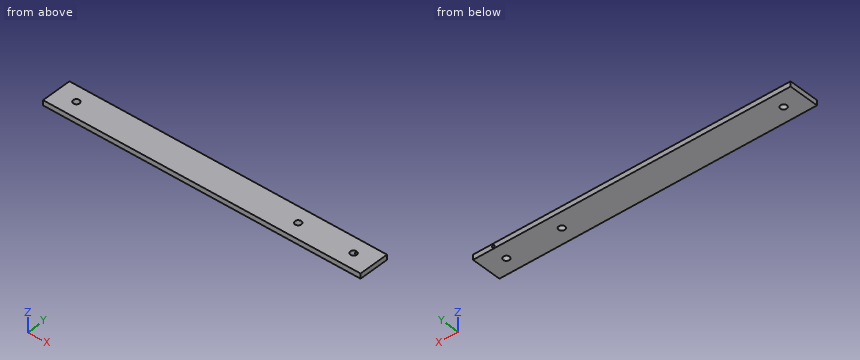
from build123d import *

# Parameters (mm, degrees)
SKETCH1_W               = 800.1
SKETCH1_H               = 76.2
BOSS_EXTRUDE1_DEPTH     = 12.7
CUT_EXTRUDE1_DEPTH      = 611.921484317
CUT_EXTRUDE1_DEPTH_BACK = 611.921484317
SKETCH2_R               = 7.9375
CUT_EXTRUDE2_DEPTH      = 615.475296493
CUT_EXTRUDE2_DEPTH_BACK = 31.75
SKETCH3_R               = 3.175


with BuildPart() as part:
    # Sketch1 → Boss-Extrude1 (new body)
    with BuildSketch(Plane.XY):
        with Locations((-209.55, 0)):
            Rectangle(SKETCH1_W, SKETCH1_H)
    extrude(amount=BOSS_EXTRUDE1_DEPTH)

    # Sketch2 → Cut-Extrude1 (cut, two sides: drawn at the far end of the back side and taken through both)
    with BuildSketch(Plane.XY.offset(12.7).offset(-CUT_EXTRUDE1_DEPTH_BACK)):
        Circle(SKETCH2_R)
        with Locations((-558.8, 0)):
            Circle(SKETCH2_R)
        with Locations((139.7, 0)):
            Circle(SKETCH2_R)
    extrude(amount=CUT_EXTRUDE1_DEPTH + CUT_EXTRUDE1_DEPTH_BACK, mode=Mode.SUBTRACT)

    # Sketch3 → Cut-Extrude2 (cut, two sides: drawn at the far end of the back side and taken through both)
    with BuildSketch(Plane(origin=(0, 38.1, 0), x_dir=(1, 0, 0), z_dir=(0, 1, 0)).offset(-CUT_EXTRUDE2_DEPTH_BACK)):
        with Locations(Location((139.7, -6.212362636, 0), (0, 0, 90))):
            Circle(SKETCH3_R)
    extrude(amount=CUT_EXTRUDE2_DEPTH + CUT_EXTRUDE2_DEPTH_BACK, mode=Mode.SUBTRACT)


solid = part.part
Could you check a few things on this model? Use its own coordinates, in mm. Coordinates: 2 decimals unless noted, no trailing zeros. Loops run counter-clockwise (first coordinate to the right, second up) from the corner with the lowest first, then second, coordinate; pieces in that order, holes last.
1. Imagine slicing it at B-B (y = 0). Please give me the cut outline in (x, z).
2. Imagine slicing it at A-A (x = -558.8). Please give me the cut outline in (y, z).
3. For P1, Ø14.5, axis at x = 139.7, y = 0, coming from the -Z side, with a flat end and sliding along its axis, tell me the tip position at first contact or that it passes through.
4. I need wall thicknesses on L1, parallel to X at y = 0, z = 5; L2, parallel to X at y = 25.5, z = 6; L3, parallel to Z at x = 139, y = 16. Which ranges of each line are inside material? Lowest first, please.
Computed values:
1. outline: (-609.6, 0) - (-566.74, 0) - (-566.74, 12.7) - (-609.6, 12.7) - close; (-550.86, 0) - (-7.94, 0) - (-7.94, 12.7) - (-550.86, 12.7) - close; (7.94, 0) - (131.76, 0) - (131.76, 12.7) - (7.94, 12.7) - close; (147.64, 0) - (190.5, 0) - (190.5, 12.7) - (147.64, 12.7) - close
2. outline: (-38.1, 0) - (-7.94, 0) - (-7.94, 12.7) - (-38.1, 12.7) - close; (7.94, 0) - (38.1, 0) - (38.1, 12.7) - (7.94, 12.7) - close
3. P1: passes through
4. L1: x = -609.6 to -566.74, -550.86 to -7.94, 7.94 to 131.76, 147.64 to 190.5
4. L2: x = -609.6 to 136.53, 142.87 to 190.5
4. L3: z = 0 to 3.12, 9.31 to 12.7
